Source: CAD feature listing. Evaluate the final solid. Frame: model axes, mm. A direction names the side the tool comes from. Round coordinates to 2 decimals unless told otherwise and drop trailing zeros. Order: outer loops, then holes, each group sorted by start corner. A loop starts at its lowest first (then second) coordinate and runs counter-clockwise, first axis right, second up. Notation, with made-up numbers: (22.5, 77) -> (77.5, 77) arc R14 ccw to (77.5, 93) -> close; hole circle Ø1 at (-4.75, -1.75). An arc over 180 degrees is marked (long way). Write item = value, one per line. Start each with the question number.
(1) Reachability of faces 4 (the face through (190, 150, 210)), 5 (the face through (208, -175, 210)), 6 (the face through (-2.45, 186.29, 823.12)), 7 (the face through (-2.45, 191.529, 872.846)) from +Z, -Z, +X, -X, +Y, -Y: full face, straight path, thin tool, end or side. Return the list, or none.
(2) Ray query, line 1 (X direction, y = -178, z = 399); line 2 (Z direction, x = -46, y = -136); line 3 (Y direction, x = -201, z = 404). Return the intervals inside material, ascending.
(3) Cut plane A-A on x = -20. Return the cut outline in (y, z).
(4) Cut plane D-D on y = 83. Return the cut outline in (x, z).
(5) Cut plane B-B on z = 513.5. Return the cut outline in (x, y), then the cut area to 3 significant figures.
(6) Contact query for flat-ended pins moving along their axis: pin 1 Ø10 at (x, y) = (-55.5, 68) entering from +Z; pin 2 Ø17.5 at (x, z) = (207, 287.5) entering from +Y; pin 3 Ø2 at (x, z) = (32, 819) entering from +Y. Output: stop coordinate, or through.
(7) Draft query along Z for faces 1 (the face through (-175, 178, 748)), 2 (the face through (3.15, 200.35, 715.82)), 3 (the face through (-225, 16, 438)). Return one class per face: released by +Z, released by -Z, zero draft, split by the parting line, or undercut.
(8) Cut plane C-C on z = 130.5. Return the cut outline in (x, y), then the cut area to 3 significant figures.
from build123d import *

# Parameters (mm, degrees)
F0_W     = 450
F0_H     = 450
F1_DEPTH = 950
F2_W     = 50
F2_H     = 50
F2_H_2   = 425
F2_W_2   = 300
F3_DEPTH = 450.001
F4_W     = 380
F4_H     = 425
F5_DEPTH = 450.001
F6_W     = 350
F6_H     = 202.6243293636
F6_H_2   = 50
F7_DEPTH = 149.1768179382


with BuildPart() as f1:
    # F0 (on Top) → F1 (new body)
    with BuildSketch(Plane.XY):
        Rectangle(F0_W, F0_H)
    extrude(amount=F1_DEPTH)

    # F2 (on face) → F3 (cut, through all)
    with BuildSketch(Plane.YZ.offset(225)):
        Polygon((-225, 475), (125, 475), (175, 950), (-225, 950), align=None)
        Polygon((175, 475), (225, 475), (225, 950), align=None)
        with Locations((200, 450)):
            Rectangle(F2_W, F2_H)
        with Locations((200, 212.5)):
            Rectangle(F2_W, F2_H_2)
        with Locations((-25, 212.5)):
            Rectangle(F2_W_2, F2_H_2)
    extrude(amount=-F3_DEPTH, mode=Mode.SUBTRACT)

    # F4 (on face) → F5 (cut, through all)
    with BuildSketch(Plane.XZ.offset(225)):
        with Locations((0, 212.5)):
            Rectangle(F4_W, F4_H)
    extrude(amount=-F5_DEPTH, mode=Mode.SUBTRACT)

    # F6 (on face) → F7 (cut, through all)
    with BuildSketch(Plane(origin=(0, 74.1780821918, -7.8082191781), x_dir=(1, 0, 0), z_dir=(0, -0.9945054529, 0.1046847845))):
        with Locations((0, 586.7878528842)):
            Rectangle(F6_W, F6_H)
        with Locations((0, 763.100017566)):
            Rectangle(F6_W, F6_H_2)
        with Locations((0, 863.100017566)):
            Rectangle(F6_W, F6_H_2)
    extrude(amount=-F7_DEPTH, mode=Mode.SUBTRACT)


solid = f1.part
Evaluation:
q1.face_4 = -Z, +Y, -Y
q1.face_5 = -Z, +X, -X
q1.face_6 = +Y
q1.face_7 = -Y
q2.line_1 = -225 to -190, 190 to 225
q2.line_2 = 425 to 475
q2.line_3 = -225 to -175, 125 to 175
q3.outline = (-225, 425) -> (175, 425) -> (175, 469.74) -> (125, 475) -> (-225, 475) -> close; (146.21, 676.51) -> (195.66, 671.31) -> (200.9, 721.03) -> (151.45, 726.24) -> close; (156.68, 775.96) -> (206.13, 770.76) -> (211.37, 820.48) -> (161.91, 825.69) -> close; (167.15, 875.41) -> (216.6, 870.21) -> (225, 950) -> (175, 950) -> close
q4.outline = (-225, 425) -> (225, 425) -> (225, 475) -> (-225, 475) -> close
q5.outline = (-225, 129.05) -> (-175, 129.05) -> (-175, 179.05) -> (-225, 179.05) -> close; (175, 129.05) -> (225, 129.05) -> (225, 179.05) -> (175, 179.05) -> close
q5.area = 5,000 mm^2
q6.pin_1 = 475
q6.pin_2 = 175
q6.pin_3 = 211.32
q7.face_1 = undercut
q7.face_2 = released by -Z
q7.face_3 = zero draft
q8.outline = (-225, -225) -> (-190, -225) -> (-190, -175) -> (-225, -175) -> close; (-225, 125) -> (-190, 125) -> (-190, 175) -> (-225, 175) -> close; (190, -225) -> (225, -225) -> (225, -175) -> (190, -175) -> close; (190, 125) -> (225, 125) -> (225, 175) -> (190, 175) -> close
q8.area = 7,000 mm^2
